Here's how the part is built. I have some questions about the finished solid (model axes, mm). Give positions to 0.01 mm unless a question says otherwise; leave off trailing zeros. Loops run counter-clockwise (first coordinate to the right, second up) from the corner with the lowest first, then second, coordinate; pieces in that order, holes last. Notation, with made-up numbers: (-4, 58.5) - (2, 58.5) arc R36 ccw to (2, 95.5) - close; hole circle Ø10 at (82.25, 82.5). An arc over 180 degrees is marked (long way). Return JSON: item names as keys, results as strings. Group by question number.
(1) I need wall thicknesses on probe 1 along Y at (x, z) = (-8, 1); probe 2 along X at (y, z) = (4.5, 1.1); probe 3 along X at (y, z) = (1, 2.85). Which ranges of each line are inside material? Lowest first, please. Write a range as [from, to].
(2) If we section it at A-A (y = 0): Please give me the cut outline in (x, z).
(3) If we section it at C-C (z = 1.3): Please give me the cut outline in (x, y), then the cut area to 3 significant figures.
(4) If we mould it in two halves opening along Y, with no side actions, what happens to faces 1 (the flat face through (12, 2, 3)), 2 (the cylindrical face through (30.238, -4.056, 1.521)), 3 (the cylindrical face through (33.579, 20.584, 1.521))? For each: released by +Y, released by -Y, zero draft, split by the parting line, or undercut.
(5) If we section it at B-B (x = -2): Please give me the cut outline in (y, z), then the cut area to 3 significant figures.
```python
from build123d import *

# Parameters (mm, degrees)
F0_W     = 56
F0_H     = 39
F0_R     = 10.5
F1_DEPTH = 3
F2_R     = 2
F3_R     = 1
F3_R_2   = 3
F4_DEPTH = 3


with BuildPart() as f1:
    # F0 (on Top) → F1 (new body)
    with BuildSketch(Plane.XY):
        with Locations((6.180598, 1.654658)):
            Rectangle(F0_W, F0_H)
        Circle(F0_R, mode=Mode.SUBTRACT)
    extrude(amount=F1_DEPTH)

    # F2
    f2_edges = [f1.edges().sort_by_distance(p)[0] for p in [
        (-21.819402, -17.845342, 1.5),
        (34.180598, -17.845342, 1.5),
        (34.180598, 21.154658, 1.5),
        (-21.819402, 21.154658, 1.5),
    ]]
    fillet(f2_edges, radius=F2_R)

    # F3 (on face) → F4 (cut, through all)
    with BuildSketch(Plane.XY.offset(3)):
        with Locations((29.314389, -3.673016)):
            Circle(F3_R)
        with Locations((14.742243, -7.630614)):
            Circle(F3_R)
        with Locations((30.968287, 8.817965)):
            Circle(F3_R)
        with Locations((21.755693, 14.060876)):
            Circle(F3_R)
        with Locations((13.471731, 16.370847)):
            Circle(F3_R)
        with Locations((6.050627, 17.455842)):
            Circle(F3_R_2)
    extrude(amount=-F4_DEPTH, mode=Mode.SUBTRACT)


solid = f1.part
```
Values:
{
 "1": {"probe 1": "[-17.85, -6.8], [6.8, 21.15]", "probe 2": "[-21.82, -9.49], [9.49, 34.18]", "probe 3": "[-21.82, -10.45], [10.45, 34.18]"},
 "2": {"outline": "(-21.82, 0) - (-10.5, 0) - (-10.5, 3) - (-21.82, 3) - close; (10.5, 0) - (34.18, 0) - (34.18, 3) - (10.5, 3) - close"},
 "3": {"outline": "(-21.82, -15.85) arc R2 ccw to (-19.82, -17.85) - (32.18, -17.85) arc R2 ccw to (34.18, -15.85) - (34.18, 19.15) arc R2 ccw to (32.18, 21.15) - (-19.82, 21.15) arc R2 ccw to (-21.82, 19.15) - close; hole circle Ø21 at (0, 0); hole circle Ø6 at (6.05, 17.46); hole circle Ø2 at (13.47, 16.37); hole circle Ø2 at (14.74, -7.63); hole circle Ø2 at (21.76, 14.06); hole circle Ø2 at (29.31, -3.67); hole circle Ø2 at (30.97, 8.82)", "area": "1,790 mm2"},
 "4": {"face 1": "zero draft", "face 2": "undercut", "face 3": "released by +Y"},
 "5": {"outline": "(-17.85, 0) - (-10.31, 0) - (-10.31, 3) - (-17.85, 3) - close; (10.31, 0) - (21.15, 0) - (21.15, 3) - (10.31, 3) - close", "area": "55.2 mm2"}
}
